Can you work these out from the drawing? Everything is in mm from the part's minimum corner. Coordinates: 2 decimals unless noted, no trailing zeros. Write each loop counter-clockwise with the first axis right and the second up, starting at its lowest first coordinate (ties: lowest second). Pieces come first, ordered by that corner, then holes.
(1) Imagine slicing it at C-C, the plane x = 106. List the corners of the cut face in (y, z) for me (3 decimals).
(2) Imagine slicing it at A-A, the plane x = 70. List the corners of the cut face in (y, z) for me (3 decimals).
(3) Imagine slicing it at D-D, the plane y = 95.5. List the corners of the cut face in (x, z) for me (3 decimals), plus the area to 3 significant figures.
(4) For pin 1 Ø1.5 at (y, z) = (83.5, 2) entering from +X; pin 2 Ø8 at (x, y) = (129.5, 70) entering from -Z, each with a flat end and sliding along its axis, tell me the tip position at first contact or that it passes through.
(5) Please list where these lines run through material, in increasing order: probe 1 along Y at (x, z) = (70, 1.35); probe 2 along Y at (x, z) = (46, 0.2); probe 3 along Y at (x, z) = (129.5, 2).
(6) Imagine slicing it at B-B, the plane z = 0.7. List the corners of the cut face in (x, y) for me, plus the area to 3 significant figures.
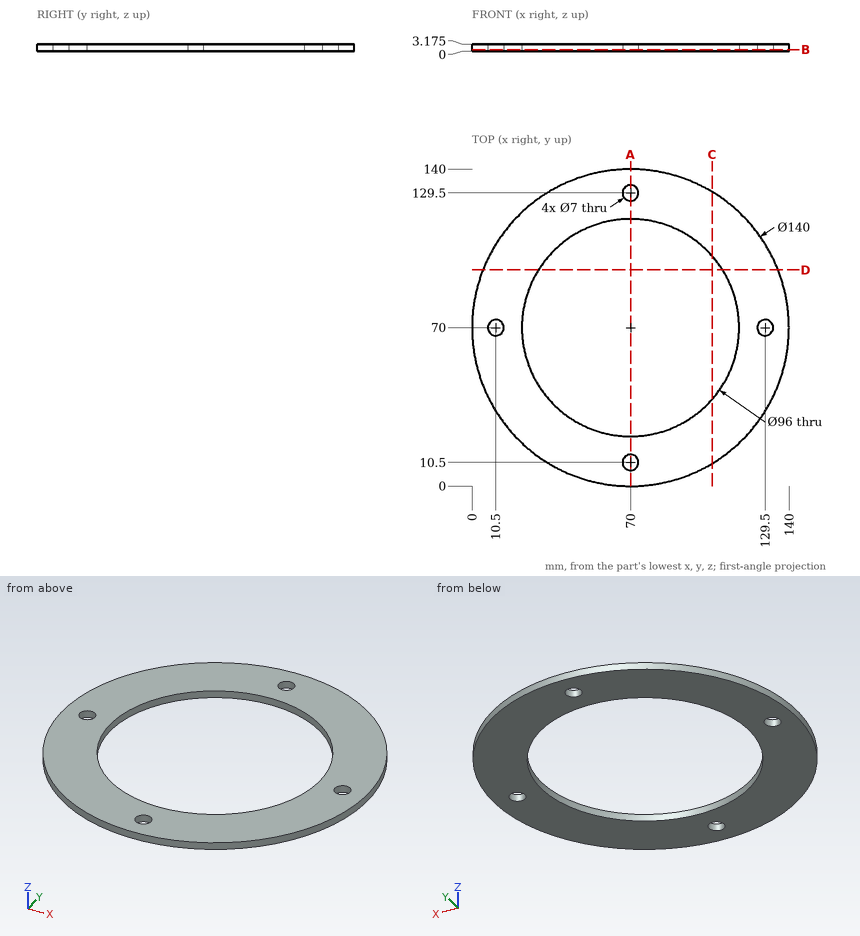
Recorded:
1. outline: (9.967, 0) - (38.251, 0) - (38.251, 3.175) - (9.967, 3.175) - close; (101.749, 0) - (130.033, 0) - (130.033, 3.175) - (101.749, 3.175) - close
2. outline: (0, 0) - (7, 0) - (7, 3.175) - (0, 3.175) - close; (14, 0) - (22, 0) - (22, 3.175) - (14, 3.175) - close; (118, 0) - (126, 0) - (126, 3.175) - (118, 3.175) - close; (133, 0) - (140, 0) - (140, 3.175) - (133, 3.175) - close
3. outline: (4.81, 0) - (29.334, 0) - (29.334, 3.175) - (4.81, 3.175) - close; (110.666, 0) - (135.19, 0) - (135.19, 3.175) - (110.666, 3.175) - close
3. area: 156 mm2
4. pin 1: stops at x = 138.83
4. pin 2: stops at z = 0
5. probe 1: y = 0 to 7, 14 to 22, 118 to 126, 133 to 140
5. probe 2: y = 4.24 to 28.43, 111.57 to 135.76
5. probe 3: y = 33.13 to 66.5, 73.5 to 106.87
6. outline: circle Ø140 at (70, 70); hole circle Ø7 at (10.5, 70); hole circle Ø96 at (70, 70); hole circle Ø7 at (70, 10.5); hole circle Ø7 at (70, 129.5); hole circle Ø7 at (129.5, 70)
6. area: 8,000 mm2
